Autodesk Fusion 360 part; units mm, degrees
sketch "Sketch1" plane through (0, 0, 0) normal (0, 0, 1) x (1, 0, 0)
sketch "Sketch2" plane through (0, 0, 0) normal (1, 0, 0) x (0, 1, 0)
  line L0 (4, 11) -> (159, 11)
  line L1 (171.5, -1.5) -> (171.5, -96.5)
  line L2 (159, -109) -> (4, -109)
  line L3 (-8.5, -96.5) -> (-8.5, -1.5)
  line L4 (0, 0) -> (163, 0)
  line L5 (163, 0) -> (163, -98)
  line L6 (163, -98) -> (0, -98)
  line L7 (0, -98) -> (0, 0)
  arc A0 (4, 11) -> (-8.5, -1.5) centre (4, -1.5) ccw
  arc A1 (171.5, -1.5) -> (159, 11) centre (159, -1.5) ccw
  arc A2 (159, -109) -> (171.5, -96.5) centre (159, -96.5) ccw
  arc A3 (-8.5, -96.5) -> (4, -109) centre (4, -96.5) ccw
  point P0 (-8.5, 11)
  point P1 (171.5, 11)
  point P2 (-8.5, -109)
  dimension "d1" = 120
  dimension "d2" = 180
  dimension "d3" = 98
  dimension "d4" = 163
  dimension "d5" = 11
  dimension "d6" = 8.5
  dimension "d13" = 12.5
extrude "Extrude1" add sketch "Sketch2" along normal blind 2
extrude "Extrude2" add 1 faces at (0, 107.3333, 3.6667) along direction (-1, 0, 0) blind 33
sketch "Sketch3" plane through (2, 0, 0) normal (1, 0, 0) x (0, 1, 0)
  line L0 (163, -98) -> (0, -98)
  line L1 (0, -98) -> (0, 0)
  line L2 (0, 0) -> (163, 0)
  line L3 (163, 0) -> (163, -98)
  line L4 (4, -109) -> (159, -109)
  line L5 (171.5, -96.5) -> (171.5, -1.5)
  line L6 (159, 11) -> (4, 11)
  line L7 (-8.5, -1.5) -> (-8.5, -96.5)
  line L8 (-8.5, -1.5) -> (159, -1.5)
  line L9 (159, -1.5) -> (159, -109)
  line L10 (159, -109) -> (-8.5, -109)
  line L11 (-8.5, -109) -> (-8.5, -1.5)
  arc A0 (4, 11) -> (-8.5, -1.5) centre (4, -1.5) ccw
  arc A1 (-8.5, -96.5) -> (4, -109) centre (4, -96.5) ccw
  arc A2 (159, -109) -> (171.5, -96.5) centre (159, -96.5) ccw
  arc A3 (171.5, -1.5) -> (159, 11) centre (159, -1.5) ccw
sketch "Sketch4" plane through (2, 0, 0) normal (1, 0, 0) x (0, 1, 0)
  line L0 (163, -98) -> (0, -98)
  line L1 (0, -98) -> (0, 0)
  line L2 (0, 0) -> (163, 0)
  line L3 (163, 0) -> (163, -98)
  arc A0 (4, 11) -> (-8.5, -1.5) centre (4, -1.5) ccw
  line L4 (-8.5, -1.5) -> (-8.5, -96.5)
  arc A1 (-8.5, -96.5) -> (4, -109) centre (4, -96.5) ccw
  line L5 (4, -109) -> (159, -109)
  arc A2 (159, -109) -> (171.5, -96.5) centre (159, -96.5) ccw
  line L6 (171.5, -96.5) -> (171.5, -1.5)
  arc A3 (171.5, -1.5) -> (159, 11) centre (159, -1.5) ccw
  line L7 (159, 11) -> (4, 11)
  line L8 (0, 0) -> (163, 0)
  line L9 (163, 0) -> (163, -98)
  line L10 (163, -98) -> (0, -98)
  line L11 (0, -98) -> (0, 0)
  line L12 (-10, 10) -> (-94.6711, 10)
  line L13 (-94.6711, 10) -> (-94.6711, 7.3388)
  line L14 (-94.6711, 7.3388) -> (-10, 7.3388)
  line L15 (-10, 7.3388) -> (-10, 10)
extrude "Extrude4" add sketch "Sketch4" along normal blind 3 contours L0 L1 L2 L3 L8 L9 L10 L11 | A0 L4 A1 L5 A2 L6 A3 L7
sketch "Sketch5" plane through (0, 0, -109) normal (0, 0, -1) x (1, 0, 0)
  line L0 (-33, -159) -> (5, -159)
  line L1 (5, -159) -> (5, -4)
  line L2 (5, -4) -> (-33, -4)
  line L3 (-33, -4) -> (-33, -159)
  circle A0 centre (-26.5, -10) radius 4
  circle A1 centre (-1.5, -10) radius 4
  circle A2 centre (-26.5, -153) radius 4
  circle A3 centre (-1.5, -153) radius 4
  dimension "d16" = 8
  dimension "d17" = 8
  dimension "d18" = 8
  dimension "d19" = 8
  dimension "d20" = 6
  dimension "d21" = 6
  dimension "d22" = 6
  dimension "d23" = 6
  dimension "d24" = 6.5
  dimension "d25" = 6.5
  dimension "d26" = 6.5
  dimension "d27" = 6.5
extrude "Extrude5" add sketch "Sketch5" along normal blind 6 contours A0 | A1 | A2 | A3
sketch "Sketch6" plane through (5, 0, 0) normal (1, 0, 0) x (0, 1, 0)
  line L0 (159, 11) -> (4, 11)
  arc A0 (4, 11) -> (-8.5, -1.5) centre (4, -1.5) ccw
  line L1 (-8.5, -1.5) -> (-8.5, -96.5)
  arc A1 (-8.5, -96.5) -> (4, -109) centre (4, -96.5) ccw
  line L2 (4, -109) -> (159, -109)
  arc A2 (159, -109) -> (171.5, -96.5) centre (159, -96.5) ccw
  line L3 (171.5, -96.5) -> (171.5, -1.5)
  arc A3 (171.5, -1.5) -> (159, 11) centre (159, -1.5) ccw
  line L4 (73, -95) -> (82, -95)
  line L5 (82, -103) -> (73, -103)
  line L6 (73, -95) -> (90, -95)
  line L7 (90, -95) -> (90, -103)
  line L8 (90, -103) -> (73, -103)
  line L9 (73, -103) -> (73, -95)
extrude "Extrude7" cut sketch "Sketch6" against normal blind 10 contours L4 L5 L6 L7 L8 L9
Build history of the part. All positions in model axes, mm. A direction names the side the tool comes from. Coordinates: 2 decimals unless noted, no trailing zeros. Write each loop counter-clockwise with the first axis right and the second up, starting at its lowest first coordinate (ties: lowest second). Pieces come first, ordered by that corner, then holes.
1. Band-saw the part on C-C, the plane y = 153. Give the cut face in (x, z), and give its area (3 significant figures).
Answer block:
outline: (-33, -109) - (-30.5, -109) - (-30.5, -115) - (-22.5, -115) - (-22.5, -109) - (-5.5, -109) - (-5.5, -115) - (2.5, -115) - (2.5, -109) - (5, -109) - (5, 11) - (-33, 11) - (-33, 0) - (2, 0) - (2, -98) - (-33, -98) - close
area: 1,230 mm2
2. Band-saw the part on B-B, the plane z = -44.5. Give the cut face in (x, y), and give its area (4 significant figures).
Answer block:
outline: (-33, -8.5) - (5, -8.5) - (5, 171.5) - (-33, 171.5) - (-33, 163) - (2, 163) - (2, 0) - (-33, 0) - close
area: 1,135 mm2
3. 3-axis set-ups, long thin cutter, end or side, ignore diameter. For faces 5 (the cylindrical face through (-30.496, 10.176, -111.958)), 6 (the flat face through (0, 73, -100)), 7 (the flat face through (-27, 153, -115)), 8 (the flat face through (-16, 83, -98)), 9 (the cylindrical face through (-14.266, 167.741, 7.435)): which of +Z, -Z, +X, -X, +Y, -Y reach the whole face in a straight line?
Answer block:
face 5: -Z
face 6: +X
face 7: -Z, +X, -X, +Y, -Y
face 8: -X
face 9: +Z, +X, -X, +Y
4. Pull direction X, two halves, no side cores. Call faces 1 (the cylindrical face through (-2.021, 13.966, -111.958)), 2 (the flat face through (0, 90, -100)), 3 (the cylindrical face through (-27.021, 156.966, -111.958)), 4 (the flat face through (-5, 81, -100)): released by +X, released by -X, zero draft, split by the parting line, or undercut.
Answer block:
face 1: undercut
face 2: zero draft
face 3: undercut
face 4: released by +X
5. Band-saw the part on A-A, the plane x = -13. Give the cut face in (y, z).
Answer block:
outline: (-8.5, -96.5) arc R12.5 ccw to (4, -109) - (159, -109) arc R12.5 ccw to (171.5, -96.5) - (171.5, -1.5) arc R12.5 ccw to (159, 11) - (4, 11) arc R12.5 ccw to (-8.5, -1.5) - close; hole (0, -98) - (163, -98) - (163, 0) - (0, 0) - close
6. Drill centre lines: probe 1 along Y at (x, z) = (-21.5, -7.5); probe 2 along Z at (x, y) = (-20, 92.5); probe 3 along Z at (x, y) = (0, 78.5). Where is each one in solid material? Low to high.
Answer block:
probe 1: y = -8.5 to 0, 163 to 171.5
probe 2: z = -109 to -98, 0 to 11
probe 3: z = -109 to -103, 0 to 11
7. Band-saw the part on D-D, the plane x = -26.5. Give the cut face in (y, z), and give its area (3 significant figures).
Answer block:
outline: (-8.5, -96.5) arc R12.5 ccw to (4, -109) - (6, -109) - (6, -115) - (14, -115) - (14, -109) - (149, -109) - (149, -115) - (157, -115) - (157, -109) - (159, -109) arc R12.5 ccw to (171.5, -96.5) - (171.5, -1.5) arc R12.5 ccw to (159, 11) - (4, 11) arc R12.5 ccw to (-8.5, -1.5) - close; hole (0, -98) - (163, -98) - (163, 0) - (0, 0) - close
area: 5,590 mm2
8. Drop flat-ended pins along their axis: pin 1 (2 mm diameter, centred on x = -26.5, y = 104.5, fed in from -Z); pin 2 (2.5 mm diameter, centred on y = 78, z = -100, fed in from +X). Give the stop position or say it passes through.
Answer block:
pin 1: stops at z = -109
pin 2: stops at x = -5
